Check sheet for the modelled part. Datum: model origin and axes. Units: mm. A direction names the side the tool comes from. Coordinates: 2 decimals unless noted, no trailing zeros. Write each loop counter-clockwise with the first axis right and the second up, starting at its lowest first coordinate (ties: lowest second). Pieces come first, ordered by that corner, then holes. Notation, with made-up numbers: (-21.5, -29) -> (-9.5, -29) arc R30 ccw to (-9.5, 3) -> close; hole circle Ø8 at (57, 66). An arc over 180 degrees is marked (long way). One line per item, written item: value. Start each with the question number.
1) Draft check along Y on faces 1 (the flat face through (0, -25.4, -21)), 2 (the flat face through (15, -50.8, 0)), 3 (the flat face through (-24.054, -25, 0)). Enter one of: +Y half, -Y half, draft (parallel to the pull), parting line (faces both ways), or undercut.
2) Sectioned sample at A-A on z = 10. Enter the section's corners in (x, y), plus the area to 3 significant figures.
3) Gauge pin test, flat ends, axial feed: P1, Ø2, axis at x = 6, y = -34, coming from the +Z side; P2, Ø4, axis at x = 12.75, z = 26.81, coming from the +Y side; P3, Ø2, axis at y = -50.5, z = -20.5, coming from the +X side. Record the tip position at first contact, or that the pin passes through.
4) Set-up check for faces 4 (the cylindrical face through (15.822, -1.507, -27.713)), 5 (the flat face through (0, -14, 8.065)), 6 (the flat face through (0, 0, 0)), 7 (the flat face through (0, -3.058, -21)): record each of +Z, -Z, +X, -X, +Y, -Y from which the full face is reachable in a straight line by a thin tool's end or side.
5) Sectioned sample at D-D on x = -12.5. Enter the section's corners in (y, z), plus the area to 3 significant figures.
6) Scan lines: line 1 along Y through (x, z) = (4, 22.5); line 2 along X through (y, z) = (-51, -5); line 3 along Y through (x, z) = (11.5, -19.5). Record each from-to range of solid material in increasing order. Write a range as [from, to].
7) Sectioned sample at C-C on z = 0. Enter the section's corners in (x, y), plus the area to 3 significant figures.
8) Sectioned sample at B-B on x = 19.5. Enter the section's corners in (y, z), plus the area to 3 significant figures.
Autodesk Inventor part; units mm, degrees
ref_plane "YZ Plane" through (0, 0, 0) normal (1, 0, 0) x (0, 1, 0)
ref_plane "XZ Plane" through (0, 0, 0) normal (0, 1, 0) x (-1, 0, 0)
ref_plane "XY Plane" through (0, 0, 0) normal (0, 0, 1) x (1, 0, 0)
sketch "Sketch10" plane through (0, 0, 0) normal (0, 1, 0) x (-1, 0, 0)
  line L0 (24.0538, -33.4645) -> (-24.0538, -33.4645)
  line L1 (-24.0538, -33.4645) -> (-24.0538, 33.4645)
  line L2 (-24.0538, 33.4645) -> (24.0538, 33.4645)
  line L3 (24.0538, 33.4645) -> (24.0538, -33.4645)
  line L4 (33.6753, 0) -> (-33.6753, 0)
  line L5 (0, -46.8503) -> (0, 46.8503)
  point P0 (0, 0)
  dimension "d17" = 66.929
  dimension "d18" = 48.1076
extrude "Extrusion4" add sketch "Sketch10" against normal blind 50.8
sketch "Sketch11" plane through (0, -50.8, 0) normal (0, -1, 0) x (1, 0, 0)
  line L0 (6.35, 25.4) -> (-6.35, 25.4)
  line L1 (-6.35, 25.4) -> (-6.35, 0)
  line L2 (-6.35, 0) -> (6.35, 0)
  line L3 (6.35, 0) -> (6.35, 25.4)
  line L4 (-33.6753, 0) -> (33.6753, 0)
  line L5 (0, -46.8503) -> (0, 46.8503)
  point P0 (0, 0)
  dimension "d21" = 25.4
  dimension "d22" = 12.7
revolve "Revolution3" add sketch "Sketch11" angle 360 about axis through (-6.35, -50.8, 0) along (1, 0, 0)
chamfer "Chamfer2" distance 25.4 angle 45 2 edges at (0, -50.8, -33.4645) (0, -50.8, 33.4645)
sketch "Sketch12" plane through (0, 0, 0) normal (0, 1, 0) x (1, 0, 0)
  circle A0 centre (12.7508, 26.7462) radius 3.2195
  line L0 (-24.0538, 33.4645) -> (24.0538, 33.4645)
  line L1 (24.0538, 33.4645) -> (24.0538, 8.0645)
  circle A1 centre (-11.2649, 26.7462) radius 3.2195
  circle A2 centre (12.7508, -26.8097) radius 3.2195
  circle A3 centre (-11.2649, -26.8097) radius 3.2195
  point P0 (0, 0)
  dimension "d27" = 6.4389
  dimension "d28" = 6.7183
  dimension "d29" = 11.303
  dimension "d32" = 24.0157
  dimension "d42" = 53.5559
  dimension "d46" = 24.0157
extrude "Extrusion5" cut sketch "Sketch12" against normal blind 5.08
sketch "Sketch13" plane through (-24.0538, 0, 33.4645) normal (0, 0, 1) x (1, 0, 0)
  line L0 (0, 0) -> (0, -25.4)
  line L1 (0, -3.0578) -> (48.1076, -3.0578)
  line L2 (48.1076, -3.0578) -> (48.1076, -25.4)
  line L3 (48.1076, -25.4) -> (0, -25.4)
  line L4 (0, -25.4) -> (0, -3.0578)
extrude "Extrusion6" cut sketch "Sketch13" against normal blind 25.4
sketch "Sketch14" plane through (24.0538, 0, -33.4645) normal (0, 0, -1) x (-1, 0, 0)
  line L0 (0, -3.0578) -> (48.1076, -3.0578)
  line L1 (48.1076, -3.0578) -> (48.1076, -25.4)
  line L2 (48.1076, -25.4) -> (0, -25.4)
  line L3 (0, -25.4) -> (0, -3.0578)
  point P0 (24.0538, 0)
extrude "Extrusion7" cut sketch "Sketch14" against normal blind 25.4
properties part number "caster wheel"
Answers:
1. face 1: undercut
1. face 2: -Y half
1. face 3: draft
2. outline: (-24.05, -48.86) -> (-6.35, -48.86) -> (-6.35, -74.15) -> (6.35, -74.15) -> (6.35, -48.86) -> (24.05, -48.86) -> (24.05, -25.4) -> (-24.05, -25.4) -> close; (-24.05, -3.06) -> (24.05, -3.06) -> (24.05, 0) -> (-24.05, 0) -> close
2. area: 1,600 mm2
3. P1: stops at z = 25.86
3. P2: stops at y = -25.4
3. P3: stops at x = 6.35
4. face 4: +Y
4. face 5: +Z, +X, -X
4. face 6: +Z, -Z, +X, -X, +Y
4. face 7: -Z, +X, -X
5. outline: (-50.8, -8.06) -> (-25.4, -33.46) -> (-25.4, -8.06) -> (-3.06, -8.06) -> (-3.06, -23.77) -> (0, -23.77) -> (0, 23.84) -> (-3.06, 23.84) -> (-3.06, 8.06) -> (-25.4, 8.06) -> (-25.4, 33.46) -> (-50.8, 8.06) -> close; (-3.06, -33.46) -> (0, -33.46) -> (0, -29.72) -> (-3.06, -29.72) -> close; (-3.06, 29.78) -> (0, 29.78) -> (0, 33.46) -> (-3.06, 33.46) -> close
5. area: 1,580 mm2
6. line 1: y = [-62.59, -39.01], [-36.36, -25.4], [-3.06, 0]
6. line 2: x = [-6.35, 6.35]
6. line 3: y = [-39.36, -25.4], [-3.06, 0]
7. outline: (-24.05, -50.8) -> (-6.35, -50.8) -> (-6.35, -76.2) -> (6.35, -76.2) -> (6.35, -50.8) -> (24.05, -50.8) -> (24.05, 0) -> (-24.05, 0) -> close
7. area: 2,770 mm2
8. outline: (-50.8, -8.06) -> (-25.4, -33.46) -> (-25.4, -8.06) -> (-3.06, -8.06) -> (-3.06, -33.46) -> (0, -33.46) -> (0, 33.46) -> (-3.06, 33.46) -> (-3.06, 8.06) -> (-25.4, 8.06) -> (-25.4, 33.46) -> (-50.8, 8.06) -> close
8. area: 1,620 mm2
